```python
from build123d import *

# Parameters (mm, degrees)
F0_R     = 70.2853794577
F0_R_2   = 16.4264849476
F0_R_3   = 14.7171878195
F1_DEPTH = 7
F2_R     = 3.49999


# Not quite as in the source:
# - a fillet or chamfer is up to 0.001 mm smaller than in the source, because OpenCascade refuses the exact size


with BuildPart() as f1:
    # F0 (on Top) → F1 (new body)
    with BuildSketch(Plane.XY):
        Circle(F0_R)
        with Locations((-35.0998191676, -20.2648900449)):
            Circle(F0_R_2, mode=Mode.SUBTRACT)
        Circle(F0_R_3, mode=Mode.SUBTRACT)
        with Locations((35.0998191676, -20.2648900449)):
            Circle(F0_R_2, mode=Mode.SUBTRACT)
        with Locations((0, 40.5297800899)):
            Circle(F0_R_2, mode=Mode.SUBTRACT)
    extrude(amount=F1_DEPTH)

    # F2 (radius 3.5 in the source; OpenCascade refuses exactly that, so slightly less here)
    f2_edges = [f1.edges().sort_by_distance(p)[0] for p in [
        (-70.285379, 0, 7),
        (-70.285379, 0, 0),
    ]]
    fillet(f2_edges, radius=F2_R)


solid = f1.part
```
CAD build for the part. Positions are in the model's coordinates, mm. Round coordinates to 2 decimals unless told otherwise and drop trailing zeros. Order: outer loops, then holes, each group sorted by start corner. A loop starts at its lowest first (then second) coordinate and runs counter-clockwise, first axis right, second up.
Item 1: Pin check, flat tips, straight feed: pin 1 (2 mm diameter, centred on x = 50, z = 6, fed in from -Y); pin 2 (2 mm diameter, centred on y = 11.5, z = 6, fed in from -X); pin 3 (1.5 mm diameter, centred on x = -35.5, z = 3, fed in from +Y). Stop position of each tip, or through.
Item 2: Mould opens along Y. For faces 1 (the face through (-1, 16, 7)), 2 (the face through (-3.19, -14.367, 3.451)) say: pulls with the +Y half, pulls with the -Y half, needs draft (parallel to the pull), parting line crosses it, or undercut.
Item 3: Probe line 1 along Y through (x, z) = (1, 4); line 2 along Y through (x, z) = (0, 4.75); line 3 along X through (y, z) = (35, 2). List the from-to ranges inside material, lowest first.
Item 4: Saw through at C-C on z = 1.25. Write the cut outline in (x, y), then the cut area to 3 significant figures.
Item 5: Saw through at B-B on x = 0. State how many separate pieces and enclosed holes the cut face has, then the cut area to 3 significant figures.
Reported:
1. pin 1: stops at y = -49.41
1. pin 2: stops at x = -69.02
1. pin 3: stops at y = 61.07
2. face 1: needs draft
2. face 2: undercut
3. line 1: y = -70.24 to -14.68, 14.68 to 24.13, 56.93 to 70.24
3. line 2: y = -70.05 to -14.72, 14.72 to 24.1, 56.96 to 70.05
3. line 3: x = -60.56 to -15.47, 15.47 to 60.56
4. outline: circle Ø138.93 at (0, 0); hole circle Ø32.85 at (-35.1, -20.26); hole circle Ø32.85 at (0, 40.53); hole circle Ø29.43 at (0, 0); hole circle Ø32.85 at (35.1, -20.26)
4. area: 11,900 mm2
5. separate pieces: 3
5. enclosed holes: 0
5. area: 537 mm2
